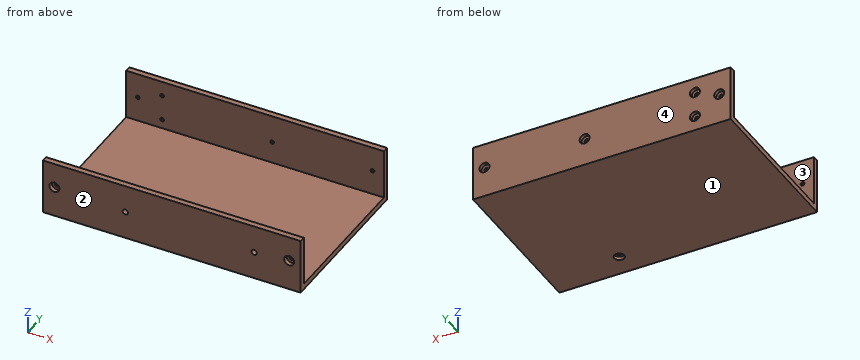
from build123d import *

# Parameters (mm, degrees)
SKICA1_W                 = 180
SKICA1_H                 = 112
P_IDAT_VYSUNUT_M1_DEPTH  = 4
SKICA3_W                 = 180
SKICA3_H                 = 4
P_IDAT_VYSUNUT_M2_DEPTH  = 35
SKICA4_R                 = 1.35
ODEBRAT_VYSUNUT_M1_DEPTH = 4
ODEBRAT_VYSUNUT_M2_REACH = 164.096
SKICA6_R                 = 1.35
SKICA7_R                 = 3.5
ODEBRAT_VYSUNUT_M3_DEPTH = 3
SKICA8_R                 = 1.85
ODEBRAT_VYSUNUT_M4_DEPTH = 4
ODEBRAT_START            = -2.5
SKICA9_R                 = 3.5
ODEBRAT_VYSUNUT_M5_DEPTH = 2.5
SKICA10_R                = 1.6
ODEBRAT_VYSUNUT_M6_DEPTH = 4
SKICA11_R                = 3.5
ODEBRAT_VYSUNUT_M7_DEPTH = 2.5


with BuildPart() as part:
    # Skica1 → Přidat vysunutím1 (new body)
    with BuildSketch(Plane.XY):
        with Locations((20.5, -3.5)):
            Rectangle(SKICA1_W, SKICA1_H)
    extrude(amount=P_IDAT_VYSUNUT_M1_DEPTH)

    # Skica3 → Přidat vysunutím2 (add)
    with BuildSketch(Plane.XY.offset(4)):
        with Locations((20.5, 50.5)):
            Rectangle(SKICA3_W, SKICA3_H)
        with Locations((20.5, -57.5)):
            Rectangle(SKICA3_W, SKICA3_H)
    extrude(amount=P_IDAT_VYSUNUT_M2_DEPTH)

    # Skica4 → Odebrat vysunutím1 (cut)
    with BuildSketch(Plane(origin=(0, 52.5, 0), x_dir=(1, 0, 0), z_dir=(0, 1, 0))):
        with Locations(Location((32.5, -19.5, 0), (0, 0, 270))):
            Circle(SKICA4_R)
        with Locations(Location((-44.5, -10.5, 0), (0, 0, 270))):
            Circle(SKICA4_R)
        with Locations(Location((-44.5, -28.5, 0), (0, 0, 270))):
            Circle(SKICA4_R)
    extrude(amount=-ODEBRAT_VYSUNUT_M1_DEPTH, mode=Mode.SUBTRACT)

    # Odebrat vysunutím2: up to this face of the body (flat: up to its plane)
    odebrat_vysunut_m2_end = Plane(part.part.faces().sort_by_distance((20.596477546, 52.5, 19.5))[0])
    # Skica6 → Odebrat vysunutím2 (cut, up to the picked face)
    with BuildSketch(Plane.XZ.offset(59.5), mode=Mode.PRIVATE) as odebrat_vysunut_m2_sk1:
        with Locations(Location((102.5, 21.5, 0), (0, 0, 270))):
            Circle(SKICA6_R)
    odebrat_vysunut_m2_tool1 = split(extrude(odebrat_vysunut_m2_sk1.sketch, amount=-ODEBRAT_VYSUNUT_M2_REACH, mode=Mode.PRIVATE), bisect_by=odebrat_vysunut_m2_end, keep=Keep.BOTH, mode=Mode.PRIVATE)
    # Skica6 → Odebrat vysunutím2 (cut, up to the picked face)
    with BuildSketch(Plane.XZ.offset(59.5), mode=Mode.PRIVATE) as odebrat_vysunut_m2_sk2:
        with Locations(Location((-61.5, 21.5, 0), (0, 0, 270))):
            Circle(SKICA6_R)
    odebrat_vysunut_m2_tool2 = split(extrude(odebrat_vysunut_m2_sk2.sketch, amount=-ODEBRAT_VYSUNUT_M2_REACH, mode=Mode.PRIVATE), bisect_by=odebrat_vysunut_m2_end, keep=Keep.BOTH, mode=Mode.PRIVATE)
    add(odebrat_vysunut_m2_tool1.solids().sort_by(Axis((102.5, -59.5, 21.5), (0, 1, 0)))[0], mode=Mode.SUBTRACT)
    add(odebrat_vysunut_m2_tool2.solids().sort_by(Axis((-61.5, -59.5, 21.5), (0, 1, 0)))[0], mode=Mode.SUBTRACT)

    # Skica7 → Odebrat vysunutím3 (cut)
    with BuildSketch(Plane.XZ.offset(59.5)):
        with Locations(Location((-61.5, 21.5, 0), (0, 0, 270))):
            Circle(SKICA7_R)
        with Locations(Location((102.5, 21.5, 0), (0, 0, 270))):
            Circle(SKICA7_R)
    extrude(amount=-ODEBRAT_VYSUNUT_M3_DEPTH, mode=Mode.SUBTRACT)

    # Skica8 → Odebrat vysunutím4 (cut)
    with BuildSketch(Plane.XZ.offset(59.5)):
        with Locations(Location((-12, 19.5, 0), (0, 0, 270))):
            Circle(SKICA8_R)
        with Locations(Location((78, 19.5, 0), (0, 0, 270))):
            Circle(SKICA8_R)
    extrude(amount=-ODEBRAT_VYSUNUT_M4_DEPTH, mode=Mode.SUBTRACT)

    # Skica9 → Odebrat vysunutím5 (cut)
    with BuildSketch(Plane(origin=(0, 52.5, 0), x_dir=(1, 0, 0), z_dir=(0, 1, 0)).offset(ODEBRAT_START)):
        with Locations(Location((-61.5, -21.5, 0), (0, 0, 90))):
            Circle(SKICA9_R)
        with Locations(Location((-44.5, -10.5, 0), (0, 0, 270))):
            Circle(SKICA9_R)
        with Locations(Location((-44.5, -28.5, 0), (0, 0, 270))):
            Circle(SKICA9_R)
        with Locations(Location((32.5, -19.5, 0), (0, 0, 270))):
            Circle(SKICA9_R)
        with Locations(Location((102.5, -21.5, 0), (0, 0, 90))):
            Circle(SKICA9_R)
    extrude(amount=ODEBRAT_VYSUNUT_M5_DEPTH, mode=Mode.SUBTRACT)

    # Skica10 → Odebrat vysunutím6 (cut)
    with BuildSketch(Plane(origin=(0, 0, 0), x_dir=(-1, 0, 0), z_dir=(0, 0, -1))):
        with Locations((-60, -43.5)):
            Circle(SKICA10_R)
    extrude(amount=-ODEBRAT_VYSUNUT_M6_DEPTH, mode=Mode.SUBTRACT)

    # Skica11 → Odebrat vysunutím7 (cut)
    with BuildSketch(Plane(origin=(0, 0, 0), x_dir=(-1, 0, 0), z_dir=(0, 0, -1))):
        with Locations((-60, -43.5)):
            Circle(SKICA11_R)
    extrude(amount=-ODEBRAT_VYSUNUT_M7_DEPTH, mode=Mode.SUBTRACT)


solid = part.part
Read the model definition and answer for the solid it produces. Units are mm, in the model's axes. Face numbers are marked on the shaded views. Give positions to 0.01 mm unless a question says otherwise; leave off trailing zeros. Loops run counter-clockwise (first coordinate to the right, second up) from the corner with the lowest first, then second, coordinate; pieces in that order, holes last. Notation, with made-up numbers: (24, 18.5) -> (28, 18.5) arc R30 cw to (28, 45.5) -> close; hole circle Ø3 at (36.25, 83.5). An arc over 180 degrees is marked (long way). Answer as CSV lines item,"result".
Item 1: Determine the mould class of the marked faces 1, 2, 3 and 4 for opening direction Y: +Y half, -Y half, draft (parallel to the pull), parting line (faces both ways), or undercut.
Returned:
face 1,"draft"
face 2,"-Y half"
face 3,"undercut"
face 4,"+Y half"
Item 2: Find section A-A on x = 78. Give the vertices of the cut face in (y, z), plus the area to 3 significant figures.
Returned:
outline,"(-59.5, 0) -> (52.5, 0) -> (52.5, 39) -> (48.5, 39) -> (48.5, 4) -> (-55.5, 4) -> (-55.5, 17.65) -> (-59.5, 17.65) -> close; (-59.5, 21.35) -> (-55.5, 21.35) -> (-55.5, 39) -> (-59.5, 39) -> close"
area,"713 mm²"
Item 3: Find section B-B on x = -2. Give the vertices of the cut face in (y, z), plus the area to 3 significant figures.
Returned:
outline,"(-59.5, 0) -> (52.5, 0) -> (52.5, 39) -> (48.5, 39) -> (48.5, 4) -> (-55.5, 4) -> (-55.5, 39) -> (-59.5, 39) -> close"
area,"728 mm²"
Item 4: Find section C-C on y = 8. Give the vertices of the cut face in (x, z), plus the area to 3 significant figures.
Returned:
outline,"(-69.5, 0) -> (110.5, 0) -> (110.5, 4) -> (-69.5, 4) -> close"
area,"720 mm²"
Item 5: Consider line 1 (Y direction, x = -42.5, z = 30); line 2 (Y direction, x = 70, z = 7); line 3 (X direction, y = 49.7, z = 28.5). Determine where each line is inside the solid, lowest interval first. Write a range as [from, to].
Returned:
line 1,"y = [-59.5, -55.5], [48.5, 50]"
line 2,"y = [-59.5, -55.5], [48.5, 52.5]"
line 3,"x = [-69.5, -45.85], [-43.15, 110.5]"
Item 6: Each of these flat-tipped pins is pushed along its axis until it touches: pin 1 (2 mm diameter, centred on x = 55.5, y = 22, fed in from +Z); pin 2 (6.5 mm diameter, centred on x = 102.5, z = 21.5, fed in from +Y). Where does it stop, or does it pass through?
Returned:
pin 1,"stops at z = 4"
pin 2,"stops at y = 50"
